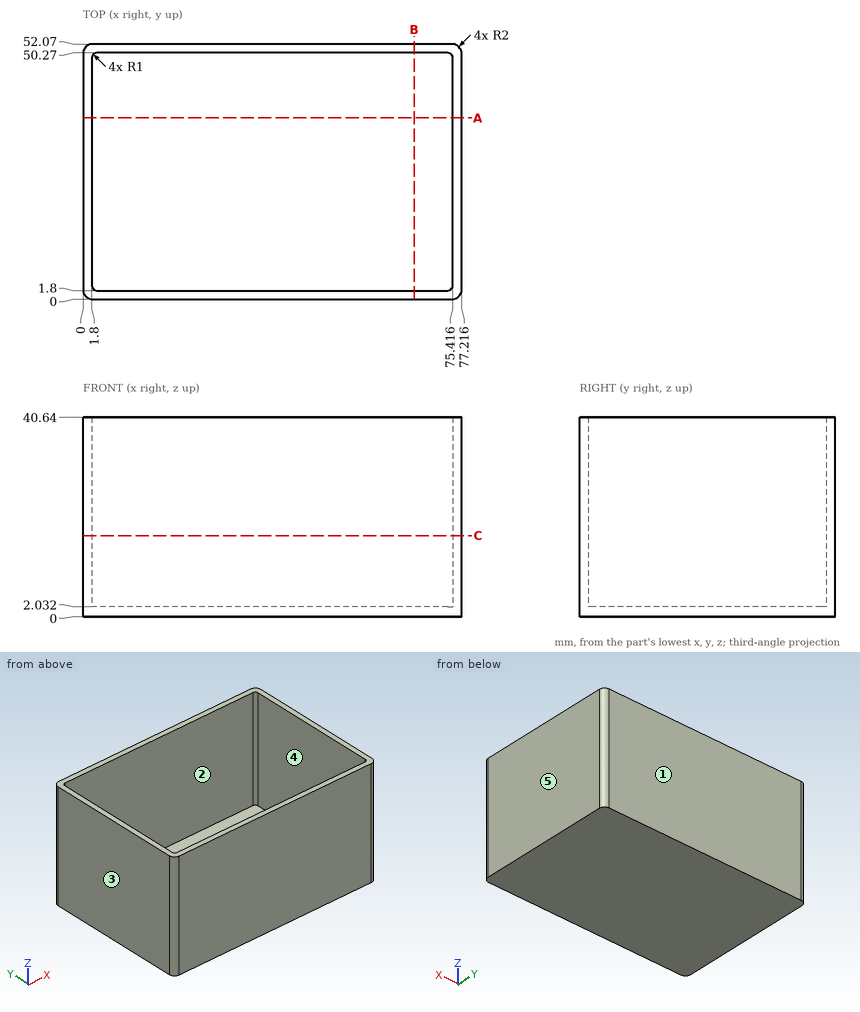
Can you work these out from the drawing? Everything is in mm from the part's minimum corner. A direction names the side the tool comes from. Coordinates: 2 decimals unless noted, no trailing zeros. Loops run counter-clockwise (first coordinate to the right, second up) from the corner with the lowest first, then second, coordinate; pieces in that order, holes last. Notation, with made-up numbers: M 4,19 L 26,19 A31 ccw 26,56 Z; hole C 13.25,44.25 d8. An arc over 180 degrees is marked long. Put each result on its own line as item: value. Start each with the question number.
(1) For the marked faces 1 and 2, which set-ups out of +Z, -Z, +X, -X, +Y, -Y let a thin tool reach every point of the face, with its end or its side?
(2) Suppose I cut it at B-B on x = 67.5. Please give me the cut outline in (y, z).
(3) Suppose I cut it at C-C on z = 16.5. Please give me the cut outline in (x, y), then the cut area to 3 significant figures.
(4) Will this pin go through, and if not, where does the flat tip stop? P1, Ø24, axis at x = 25, y = 29.5, coming from the +Z side.
(5) I need wall thicknesses on line 1 (Y direction, x = 54.5, z = 22); line 2 (X direction, y = 34, z = 9); line 3 (Z direction, x = 9, y = 32.5). Which ranges of each line are inside material? Lowest first, please. Write a range as from..to.
(6) Suppose I cut it at A-A on y = 37. Please give me the cut outline in (x, z), then the cut area to 3 significant figures.
(7) Thinking about a two-plate mould opening in X: for the marked faces 3, 4 and 5, which applies, pulls with the +X half, pulls with the -X half, needs draft (parallel to the pull), parting line crosses it, or undercut?
Solutions:
1. face 1: +Z, -Z, +X, -X, +Y
1. face 2: +Z
2. outline: M 0,0 L 52.07,0 L 52.07,40.64 L 50.27,40.64 L 50.27,2.03 L 1.8,2.03 L 1.8,40.64 L 0,40.64 Z
3. outline: M 0,2 A2 ccw 2,0 L 75.22,0 A2 ccw 77.22,2 L 77.22,50.07 A2 ccw 75.22,52.07 L 2,52.07 A2 ccw 0,50.07 Z; hole M 1.8,2.8 A1 ccw 2.8,1.8 L 74.42,1.8 A1 ccw 75.42,2.8 L 75.42,49.27 A1 ccw 74.42,50.27 L 2.8,50.27 A1 ccw 1.8,49.27 Z
3. area: 450 mm2
4. P1: stops at z = 2.03
5. line 1: y = 0..1.8, 50.27..52.07
5. line 2: x = 0..1.8, 75.42..77.22
5. line 3: z = 0..2.03
6. outline: M 0,0 L 77.22,0 L 77.22,40.64 L 75.42,40.64 L 75.42,2.03 L 1.8,2.03 L 1.8,40.64 L 0,40.64 Z
6. area: 296 mm2
7. face 3: pulls with the -X half
7. face 4: undercut
7. face 5: pulls with the +X half
